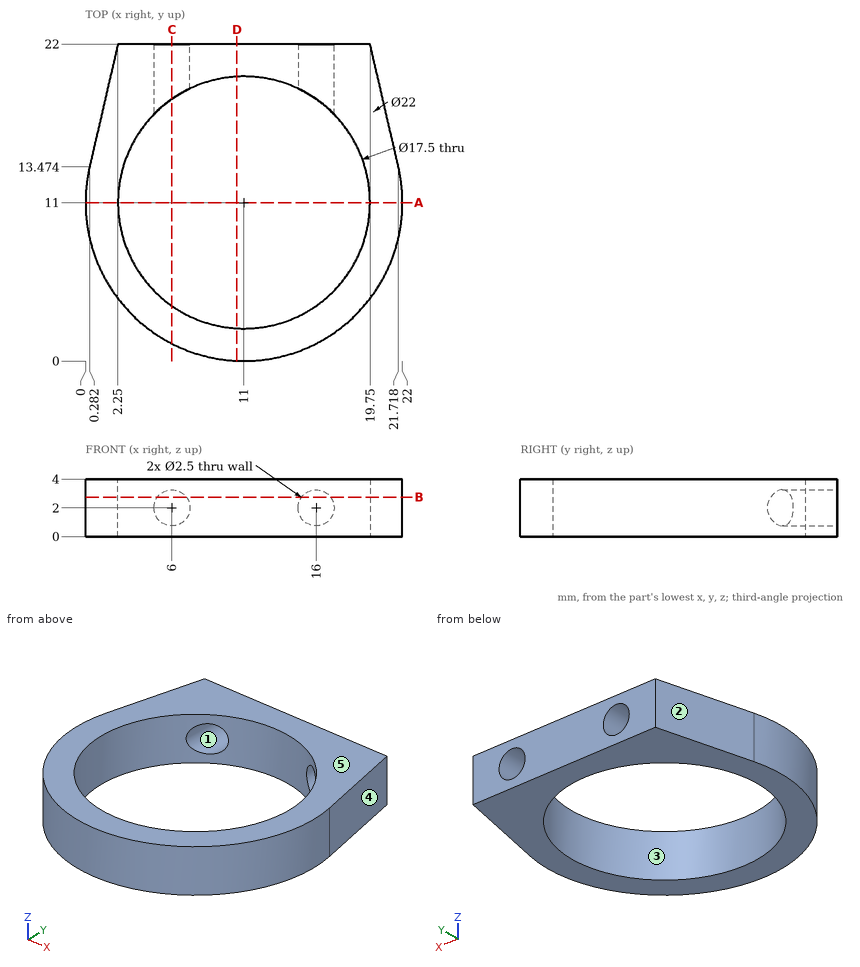
Geometry: see drawing. Coordinates: mm, zero at the bounding-box minimum. A direction names the side the tool comes from. Coordinates: 2 decimals unless noted, no trailing zeros. Order: outer loops, then holes, each group sorted by start corner. A loop starts at its lowest first (then second) coordinate and runs counter-clockwise, first axis right, second up. Notation, with made-up numbers: M 71.5,5 L 127.5,5 A13 ccw 127.5,28 Z; hole C 58.5,22.25 d5. An arc over 180 degrees is marked long. Answer as CSV lines item,"result".
1. Section B-B (z = 2.75). Return the cut outline in (x, y), then the cut area to 3 significant figures.
Reported:
outline,"M 0.28,13.47 A11 ccw long 21.72,13.47 L 19.75,22 L 17,22 L 17,17.37 A8.75 cw long 5,17.37 L 5,22 L 2.25,22 Z; M 7,18.78 A8.75 cw 15,18.78 L 15,22 L 7,22 Z"
area,"154 mm2"
2. Section C-C (x = 6). Return the cut outline in (y, z).
Reported:
outline,"M 1.2,0 L 3.82,0 L 3.82,4 L 1.2,4 Z; M 18.18,0 L 22,0 L 22,0.75 L 18.18,0.75 Z; M 18.18,3.25 L 22,3.25 L 22,4 L 18.18,4 Z"
3. Material intervals for line 1 (Y direction, x = 10.75, z = 0.9); line 2 (Z direction, x = 6, y = 18.6); line 3 (Y direction, x = 9.5, z = 0.95), sorted ascending. Write a range as from..to.
Reported:
line 1,"0..2.25, 19.75..22"
line 2,"0..0.75, 3.25..4"
line 3,"0.1..2.38, 19.62..22"
4. Section A-A (y = 11). Return the cut outline in (x, z).
Reported:
outline,"M 0,0 L 2.25,0 L 2.25,4 L 0,4 Z; M 19.75,0 L 22,0 L 22,4 L 19.75,4 Z"
5. Section D-D (x = 10.5). Return the cut outline in (y, z), then the cut area to 3 significant figures.
Reported:
outline,"M 0.01,0 L 2.26,0 L 2.26,4 L 0.01,4 Z; M 19.74,0 L 22,0 L 22,4 L 19.74,4 Z"
area,"18.1 mm2"
6. Access query for the marked faces 1 and 2. Directions: +Z, -Z, +X, -X, +Y, -Y. A direction counts if a zero-diameter tool reaches every point of the face in a straight line with its end or side. Return the directions, or none.
Reported:
face 1,"+Y"
face 2,"+Z, -Z, -X, +Y"
7. First-contact query: P1, Ø10, axis at x = 17, y = 6.5, coming from the -Z side; P2, Ø1.5, axis at y = 8, z = 2, coming from the +X side; P3, Ø1, axis at y = 14.5, z = 2.5, coming from the +X side. Flat tips, straight axial feed; report the tip coordinate or a pass-through.
Reported:
P1,"z = 0"
P2,"x = 21.77"
P3,"x = 21.6"
8. Pull-direction query (X, two-part tool) for the marked faces 3, 4 and 5; classes: released by +X, released by -X, zero draft, split by the parting line, or undercut.
Reported:
face 3,"undercut"
face 4,"released by +X"
face 5,"zero draft"
